from build123d import *

# Parameters (mm, degrees)
SKETCH1_R           = 35
BOSS_EXTRUDE1_DEPTH = 5
SKETCH3_R           = 37.5
BOSS_EXTRUDE2_DEPTH = 5
SKETCH4_R           = 27.5
BOSS_EXTRUDE5_DEPTH = 116
SKETCH5_R           = 32.5
BOSS_EXTRUDE6_DEPTH = 5
SKETCH6_R           = 30
BOSS_EXTRUDE7_DEPTH = 3
FILLET1_R           = 10
FILLET2_R           = 10


with BuildPart() as part:
    # Sketch1 → Boss-Extrude1 (new body)
    with BuildSketch(Plane(origin=(0, 0, 0), x_dir=(1, 0, 0), z_dir=(0, 1, 0))):
        with Locations(Location((0, 0, 0), (0, 0, 270))):
            Circle(SKETCH1_R)
    extrude(amount=BOSS_EXTRUDE1_DEPTH)

    # Sketch3 → Boss-Extrude2 (add)
    with BuildSketch(Plane(origin=(0, 5, 0), x_dir=(1, 0, 0), z_dir=(0, 1, 0))):
        with Locations(Location((0, 0, 0), (0, 0, 270))):
            Circle(SKETCH3_R)
    extrude(amount=BOSS_EXTRUDE2_DEPTH)

    # Sketch4 → Boss-Extrude5 (add)
    with BuildSketch(Plane(origin=(0, 10, 0), x_dir=(1, 0, 0), z_dir=(0, 1, 0))):
        with Locations(Location((0, 0, 0), (0, 0, 90))):
            Circle(SKETCH4_R)
    extrude(amount=BOSS_EXTRUDE5_DEPTH)

    # Sketch5 → Boss-Extrude6 (add)
    with BuildSketch(Plane(origin=(0, 126, 0), x_dir=(1, 0, 0), z_dir=(0, 1, 0))):
        with Locations(Location((0, 0, 0), (0, 0, 270))):
            Circle(SKETCH5_R)
    extrude(amount=BOSS_EXTRUDE6_DEPTH)

    # Sketch6 → Boss-Extrude7 (add)
    with BuildSketch(Plane(origin=(0, 131, 0), x_dir=(1, 0, 0), z_dir=(0, 1, 0))):
        with Locations(Location((0, 0, 0), (0, 0, 270))):
            Circle(SKETCH6_R)
    extrude(amount=BOSS_EXTRUDE7_DEPTH)

    # Fillet1
    # the kernel refuses this fillet: 10 mm, written as the material it adds along each edge
    with BuildSketch(Plane(origin=(0, 10, 0), x_dir=(0, 0, -1), z_dir=(1, 0, 0))) as fillet1_piece_1:
        with BuildLine():
            CenterArc((27.5 + FILLET1_R, FILLET1_R), FILLET1_R, 180, 90)
            Line((27.5 + FILLET1_R, 0), (27.5 + FILLET1_R, -FILLET1_R * 0.02))
            Line((27.5 + FILLET1_R, -FILLET1_R * 0.02), (27.5 - FILLET1_R * 0.02, -FILLET1_R * 0.02))
            Line((27.5 - FILLET1_R * 0.02, -FILLET1_R * 0.02), (27.5 - FILLET1_R * 0.02, FILLET1_R))
            Line((27.5 - FILLET1_R * 0.02, FILLET1_R), (27.5, FILLET1_R))
        make_face()
    revolve(axis=Axis((0, 10, 0), (0, 1, 0)))
    with BuildSketch(Plane(origin=(0, 126, 0), x_dir=(0, 0, -1), z_dir=(1, 0, 0))) as fillet1_piece_2:
        with BuildLine():
            CenterArc((37.5, -8.660254038), FILLET1_R, 120, 60)
            Line((27.5, -8.660254038), (27.3, -8.660254038))
            Line((27.3, -8.660254038), (27.3, 0))
            Line((27.3, 0), (27.5, 0.2))
            ThreePointArc((27.5, 0.2), (30, 0.2), (32.4, 0.173205081))
            Line((32.4, 0.173205081), (32.5, 0))
        make_face()
    revolve(axis=Axis((0, 126, 0), (0, 1, 0)))

    # Fillet2
    # the kernel refuses this fillet: 10 mm, written as the material it takes off along each edge
    with BuildSketch(Plane(origin=(0, 126, 0), x_dir=(0, 0, 1), z_dir=(-1, 0, 0))) as fillet2_piece_1:
        with BuildLine():
            CenterArc((22.5, 4.568502517), FILLET2_R, 318.590377891, 41.409622109)
            Line((32.5, 4.568502517), (32.7, 4.568502517))
            Line((32.7, 4.568502517), (32.7, 0))
            Line((32.7, 0), (32.6, -0.173205081))
            ThreePointArc((32.6, -0.173205081), (31.293504258, -1.076098804), (30.15, -2.178163326))
            Line((30.15, -2.178163326), (30, -2.04587576))
        make_face()
    revolve(axis=Axis((0, 126, 0), (0, 1, 0)), revolution_arc=180, mode=Mode.SUBTRACT)
    with BuildSketch(Plane(origin=(0, 10, 0), x_dir=(0, 0, -1), z_dir=(1, 0, 0))) as fillet2_piece_2:
        with BuildLine():
            CenterArc((27.817541634, -7.5), FILLET2_R, 14.477512186, 46.567463442)
            Line((37.5, -5), (37.693649167, -4.95))
            ThreePointArc((37.693649167, -4.95), (37.7, -2.5), (37.7, 0))
            Line((37.7, 0), (37.5, 0.2))
            ThreePointArc((37.5, 0.2), (35.05, 0.511190802), (32.755595401, 1.425))
            Line((32.755595401, 1.425), (32.658770817, 1.25))
        make_face()
    revolve(axis=Axis((0, 10, 0), (0, 1, 0)), revolution_arc=180, mode=Mode.SUBTRACT)
    with BuildSketch(Plane(origin=(0, 10, 0), x_dir=(0, 0, 1), z_dir=(-1, 0, 0))) as fillet2_piece_3:
        with BuildLine():
            CenterArc((27.817541634, -7.5), FILLET2_R, 14.477512186, 46.567463442)
            Line((37.5, -5), (37.693649167, -4.95))
            ThreePointArc((37.693649167, -4.95), (37.7, -2.5), (37.7, 0))
            Line((37.7, 0), (37.5, 0.2))
            ThreePointArc((37.5, 0.2), (35.05, 0.511190802), (32.755595401, 1.425))
            Line((32.755595401, 1.425), (32.658770817, 1.25))
        make_face()
    revolve(axis=Axis((0, 10, 0), (0, 1, 0)), revolution_arc=180, mode=Mode.SUBTRACT)
    with BuildSketch(Plane(origin=(0, 126, 0), x_dir=(0, 0, -1), z_dir=(1, 0, 0))) as fillet2_piece_4:
        with BuildLine():
            CenterArc((22.5, 4.568502517), FILLET2_R, 318.590377891, 41.409622109)
            Line((32.5, 4.568502517), (32.7, 4.568502517))
            Line((32.7, 4.568502517), (32.7, 0))
            Line((32.7, 0), (32.6, -0.173205081))
            ThreePointArc((32.6, -0.173205081), (31.293504258, -1.076098804), (30.15, -2.178163326))
            Line((30.15, -2.178163326), (30, -2.04587576))
        make_face()
    revolve(axis=Axis((0, 126, 0), (0, 1, 0)), revolution_arc=180, mode=Mode.SUBTRACT)


solid = part.part
Check sheet for the modelled part. Datum: model origin and axes. Units: mm. A direction names the side the tool comes from. Give positions to 0.01 mm unless a question says otherwise; leave off trailing zeros. Loops run counter-clockwise (first coordinate to the right, second up) from the corner with the lowest first, then second, coordinate; pieces in that order, holes last. Notation, with made-up numbers: M -2.75,82 L 7.25,82 A12 cw 7.25,97 Z; hole C 57.25,34.25 d6. An arc over 180 degrees is marked long. Return JSON: item names as keys, results as strings. Group by question number.
1. Cross-section at D-D on y = 17.5. Record the boundary of the cut face in (x, z), plus the area to 3 significant figures.
2. Go/stop test with flat-tipped pins: pin 1 (6 mm diameter, centred on x = 15, y = 69, fed in from -Z); pin 2 (10 mm diameter, centred on y = 90, z = 26.5, fed in from -X); pin 3 (2 mm diameter, centred on x = 4, y = 44, fed in from -Z). Record where each tip stops, or that it passes through.
3. Mould release check, pull along Y, two halves, no side actions. Record for faces 1 (the flat face through (17, 5, -31)), 2 (the flat face through (-29, 131, 9)), 3 (the cylindrical face through (-21, 2, -28)), 4 (the cylindrical face through (24.397, 67.988, -12.69)): released by +Y, released by -Y, zero draft, split by the parting line, or undercut.
4. Cross-section at C-C on y = 37.5. Record the boundary of the cut face in (x, z).
5. Cross-section at B-B on z = 0. Record the boundary of the cut face in (x, y).
6. Cross-section at A-A on x = 0. Record the boundary of the cut face in (y, z), plus the area to 3 significant figures.
7. Tool access check on faces 5 (the cylindrical face through (9.76, 130.78, 31)), 6 (the flat face through (0, 0, 0)). Record the directions out of +Z, -Z, +X, -X, +Y, -Y that give a thin tool (end or side, any length) a straight path to the whole face; none if there is none.
8. Thickness scan on L1, parallel to Y at x = -29, z = -11; L2, parallel to Y at x = -28.5, z = -2.5; L3, parallel to X at y = 76.5, z = 0.5. Record the ranges inside material, lowest first.
Return value:
{
 "1": {"outline": "C 0,0 d55.64", "area": "2,430 mm^2"},
 "2": {"pin 1": "z = -24.74", "pin 2": "x = -17.15", "pin 3": "z = -27.34"},
 "3": {"face 1": "released by -Y", "face 2": "released by +Y", "face 3": "zero draft", "face 4": "undercut"},
 "4": {"outline": "C 0,0 d55"},
 "5": {"outline": "M -37.5,5 L -35,5 L -35,0 L 35,0 L 35,5 L 37.5,5 A10 ccw 32.66,11.25 A10 cw 27.5,20 L 27.5,117.34 A10 cw 30,123.95 A10 ccw 32.5,130.57 L 32.5,131 L 30,131 L 30,134 L -30,134 L -30,131 L -32.5,131 L -32.5,130.57 A10 ccw -30,123.95 A10 cw -27.5,117.34 L -27.5,20 A10 cw -32.66,11.25 A10 ccw Z"},
 "6": {"outline": "M 0,-35 L 5,-35 L 5,-37.5 A10 ccw 11.25,-32.66 A10 cw 20,-27.5 L 117.34,-27.5 A10 cw 123.95,-30 A10 ccw 130.57,-32.5 L 131,-32.5 L 131,-30 L 134,-30 L 134,30 L 131,30 L 131,32.5 L 130.57,32.5 A10 ccw 123.95,30 A10 cw 117.34,27.5 L 20,27.5 A10 cw 11.25,32.66 A10 ccw 5,37.5 L 5,35 L 0,35 Z", "area": "7,660 mm^2"},
 "7": {"face 5": "+Y", "face 6": "+Z, -Z, +X, -X, -Y"},
 "8": {"L1": "0 to 12.39, 125.33 to 131", "L2": "0 to 15.42, 121.92 to 134", "L3": "-27.5 to 27.5"}
}
